Read the model definition and answer for the solid it produces. Units are mm, in the model's axes. Face numbers are marked on the shaded views. A direction names the side the tool comes from. Give positions to 0.01 mm unless a question says otherwise; leave off trailing zeros. Order: outer loops, then holes, each group sorted by start corner. A loop starts at its lowest first (then second) coordinate and runs counter-clockwise, first axis right, second up. Notation, with made-up numbers: (53, 76.25) - (73, 76.25) arc R30 ccw to (73, 104.25) - close; hole circle Ø11 at (51.25, -33). An arc over 180 degrees is marked (long way). Write each question's results on one line, items separated by ' | '.
from build123d import *

# Parameters (mm, degrees)
F1_DEPTH = 2
F3_DEPTH = 20
F5_DEPTH = 12.5


# Not quite as in the source:
# - a feature names something its author has since deleted; it is built from what else it names


with BuildPart() as f1:
    # F0 (on Front) → F1 (new body)
    with BuildSketch(Plane.XZ):
        with BuildLine():
            Line((79.8777135909, 45.9989449601), (-67.1222864091, 45.9989449601))
            ThreePointArc((-67.1222864091, 45.9989449601), (-69.9507135339, 44.8273720848), (-71.1222864091, 41.9989449601))
            Line((-71.1222864091, 41.9989449601), (-71.1222864091, -32.0010550399))
            ThreePointArc((-71.1222864091, -32.0010550399), (-69.9507135339, -34.8294821647), (-67.1222864091, -36.0010550399))
            Line((-67.1222864091, -36.0010550399), (79.8777135909, -36.0010550399))
            ThreePointArc((79.8777135909, -36.0010550399), (82.7061407156, -34.8294821647), (83.8777135909, -32.0010550399))
            Line((83.8777135909, -32.0010550399), (83.8777135909, 41.9989449601))
            ThreePointArc((83.8777135909, 41.9989449601), (82.7061407156, 44.8273720848), (79.8777135909, 45.9989449601))
        make_face()
    extrude(amount=F1_DEPTH)

    # F2 (on face) → F3 (join)
    with BuildSketch(Plane.XZ.offset(2)):
        with BuildLine():
            ThreePointArc((83.8777135909, 41.9989449601), (82.7061407156, 44.8273720848), (79.8777135909, 45.9989449601))
            Line((79.8777135909, 45.9989449601), (-67.1222864091, 45.9989449601))
            ThreePointArc((-67.1222864091, 45.9989449601), (-69.9507135339, 44.8273720848), (-71.1222864091, 41.9989449601))
            Line((-71.1222864091, 41.9989449601), (-71.1222864091, -32.0010550399))
            ThreePointArc((-71.1222864091, -32.0010550399), (-69.9507135339, -34.8294821647), (-67.1222864091, -36.0010550399))
            Line((-67.1222864091, -36.0010550399), (79.8777135909, -36.0010550399))
            ThreePointArc((79.8777135909, -36.0010550399), (82.7061407156, -34.8294821647), (83.8777135909, -32.0010550399))
            Line((83.8777135909, -32.0010550399), (83.8777135909, 41.9989449601))
        make_face()
        with BuildLine():
            ThreePointArc((-69.6222864091, 40.4989449601), (-68.4507135339, 43.3273720848), (-65.6222864091, 44.4989449601))
            Line((-65.6222864091, 44.4989449601), (78.3777135909, 44.4989449601))
            ThreePointArc((78.3777135909, 44.4989449601), (81.2061407156, 43.3273720848), (82.3777135909, 40.4989449601))
            Line((82.3777135909, 40.4989449601), (82.3777135909, -30.5010550399))
            ThreePointArc((82.3777135909, -30.5010550399), (81.2061407156, -33.3294821647), (78.3777135909, -34.5010550399))
            Line((78.3777135909, -34.5010550399), (-65.6222864091, -34.5010550399))
            ThreePointArc((-65.6222864091, -34.5010550399), (-68.4507135339, -33.3294821647), (-69.6222864091, -30.5010550399))
            Line((-69.6222864091, -30.5010550399), (-69.6222864091, 40.4989449601))
        make_face(mode=Mode.SUBTRACT)
    extrude(amount=F3_DEPTH)

    # F4 (on face) → F5 (cut, symmetric)
    with BuildSketch(Plane.XZ.offset(2)):
        Polygon((14.3804825891, 28.8355327559), (10.8255747657, 35.7375912952), (3.0707628205, 36.1099800817), (-1.1291413013, 29.5803103289), (2.4257665221, 22.6782517895), (10.1805784673, 22.305863003), align=None)
        Polygon((35.2220927825, 16.5163073577), (31.6671849591, 23.4183658971), (23.9123730139, 23.7907546836), (19.7124688921, 17.2610849307), (23.2673767155, 10.3590263914), (31.0221886607, 9.9866376049), align=None)
        Polygon((30.7742316076, -14.2223389774), (34.9741357295, -7.6926692246), (31.419227906, -0.7906106852), (23.6644159608, -0.4182218987), (19.464511839, -6.9478916516), (23.0194196624, -13.8499501909), align=None)
        Polygon((1.929852416, -25.7397013751), (9.6846643612, -26.1120901616), (13.884568483, -19.5824204088), (10.3296606596, -12.6803618694), (2.5748487144, -12.3079730829), (-1.6250554074, -18.8376428357), align=None)
        Polygon((-22.4666656008, -6.5184174376), (-18.9117577774, -13.420475977), (-11.1569458322, -13.7928647635), (-6.9570417103, -7.2631950106), (-10.5119495338, -0.3611364712), (-18.266761479, 0.0112523153), align=None)
        Polygon((-18.0188044259, 24.2202288976), (-22.2187085477, 17.6905591447), (-18.6638007243, 10.7885006053), (-10.9089887791, 10.4161118188), (-6.7090846573, 16.9457815717), (-10.2639924807, 23.8478401111), align=None)
        Polygon((2.1058970544, -2.4000583217), (10.6495301273, -2.4000583217), (14.9213466637, 4.9989449601), (10.6495301273, 12.3979482418), (2.1058970544, 12.3979482418), (-2.165919482, 4.9989449601), align=None)
    extrude(amount=F5_DEPTH, both=True, mode=Mode.SUBTRACT)


solid = f1.part
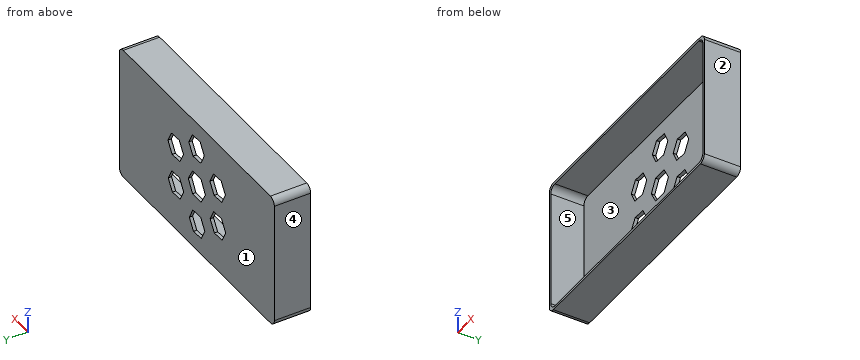
(1) Each of these flat-tipped pins is pushed along its axis until it touches: pin 1 (8 mm diameter, centred on x = 47.5, z = -12, fed in from +Y); pin 2 (6 mm diameter, centred on x = 64, z = 17, fed in from -Y). Where does it stop, or does it pass through?
Conclusion:
pin 1: y = 0 | pin 2: y = -2
(2) The mould has two halves that part along X. Classify the marked faces 1, 2 and 3: pulls with the +X half, pulls with the -X half, needs draft (parallel to the pull), parting line crosses it, or undercut.
Conclusion:
face 1: needs draft | face 2: pulls with the +X half | face 3: undercut
(3) For the marked faces 4 and 5, determine the directions among +Z, -Z, +X, -X, +Y, -Y from which every point of the face is accessible in a straight line to the end or side of a thin tool.
Conclusion:
face 4: +Z, -Z, -X, +Y, -Y | face 5: -Y
(4) Section C-C (x = -57) is taken. Give the vertices of the cut face in (y, z).
Conclusion:
outline: (-22, -36) - (0, -36) - (0, 46) - (-22, 46) - (-22, 44.5) - (-2, 44.5) - (-2, -34.5) - (-22, -34.5) - close
(5) Section A-A (y = -16) is taken. Give the vertices of the cut face in (x, z).
Conclusion:
outline: (-71.12, -32) arc R4 ccw to (-67.12, -36) - (79.88, -36) arc R4 ccw to (83.88, -32) - (83.88, 42) arc R4 ccw to (79.88, 46) - (-67.12, 46) arc R4 ccw to (-71.12, 42) - close; hole (-69.62, -30.5) arc R4 ccw to (-65.62, -34.5) - (78.38, -34.5) arc R4 ccw to (82.38, -30.5) - (82.38, 40.5) arc R4 ccw to (78.38, 44.5) - (-65.62, 44.5) arc R4 ccw to (-69.62, 40.5) - close
(6) Section B-B (z = 32.5) is taken. Give the vertices of the cut face in (x, y), plus the area to 3 significant figures.
Conclusion:
outline: (-71.12, -22) - (-69.62, -22) - (-69.62, -2) - (0.75, -2) - (0.75, 0) - (-71.12, 0) - close; (12.49, -2) - (82.38, -2) - (82.38, -22) - (83.88, -22) - (83.88, 0) - (12.49, 0) - close | area: 347 mm^2
(7) Consider probe 1 along X at (y, z) = (-4.75, -2.5); probe 2 along Z at (x, y) = (-65, -9.5); probe 3 along X at (y, z) = (-0.75, 16.5). Determine where each line is inside the solid, lowest interval first. Write a range as [from, to].
Conclusion:
probe 1: [-71.12, -69.62], [82.38, 83.88] | probe 2: [-36, -34.5], [44.5, 46] | probe 3: [-71.12, -21.61], [-7, 20.1], [35.21, 83.88]
